CAD build for the part. Positions are in the model's coordinates, mm. Coordinates: 2 decimals unless noted, no trailing zeros. Order: outer loops, then holes, each group sorted by start corner. A loop starts at its lowest first (then second) coordinate and runs counter-clockwise, first axis right, second up. Notation, with made-up numbers: (-31.75, -22) - (-14.75, -22) arc R13 cw to (-14.75, 0) - close; hole circle Ø1 at (41, -24). An arc over 180 degrees is marked (long way). Return JSON: item names as keys, results as strings.
from build123d import *

# Parameters (mm, degrees)
SKETCH2_R           = 9.525
SKETCH2_R_2         = 8.5725
BOSS_EXTRUDE1_DEPTH = 3.175
BOSS_EXTRUDE2_DEPTH = 3.175
BOSS_EXTRUDE3_DEPTH = 10.16
SKETCH5_R           = 1.4351
CUT_EXTRUDE1_DEPTH  = 19.05


with BuildPart() as part:
    # Sketch2 → Boss-Extrude1 (new body, symmetric)
    with BuildSketch(Plane(origin=(0, 0, 0), x_dir=(1, 0, 0), z_dir=(0, 1, 0))):
        Circle(SKETCH2_R)
        Circle(SKETCH2_R_2, mode=Mode.SUBTRACT)
    extrude(amount=BOSS_EXTRUDE1_DEPTH, both=True)

    # Sketch3 → Boss-Extrude2 (add, symmetric)
    with BuildSketch(Plane(origin=(0, 0, 0), x_dir=(1, 0, 0), z_dir=(0, 1, 0))):
        with BuildLine():
            Line((-9.525, 0), (-9.525, -16.764))
            ThreePointArc((-9.525, -16.764), (0, -17.294810057), (9.525, -16.764))
            Line((9.525, -16.764), (9.525, 0))
            ThreePointArc((9.525, 0), (0, -9.525), (-9.525, 0))
        make_face()
    extrude(amount=BOSS_EXTRUDE2_DEPTH, both=True)

    # Sketch4 → Boss-Extrude3 (add)
    with BuildSketch(Plane(origin=(0, 0, 0), x_dir=(1, 0, 0), z_dir=(0, 1, 0))):
        with BuildLine():
            Line((-9.525, -16.764), (-9.525, -13.716))
            Line((-9.525, -13.716), (9.525, -13.716))
            Line((9.525, -13.716), (9.525, -16.764))
            ThreePointArc((9.525, -16.764), (0, -17.294810057), (-9.525, -16.764))
        make_face()
    extrude(amount=BOSS_EXTRUDE3_DEPTH)

    # Sketch5 → Cut-Extrude1 (cut)
    with BuildSketch(Plane(origin=(0, 0, 13.716), x_dir=(-1, 0, 0), z_dir=(0, 0, -1))):
        with Locations((0, 6.6675)):
            Circle(SKETCH5_R)
    extrude(amount=-CUT_EXTRUDE1_DEPTH, mode=Mode.SUBTRACT)


solid = part.part
Item 1: Band-saw the part on A-A, the plane x = 0. List the corners of the cut face in (y, z) (1 decimal), then the cut area to 3 significant figures.
Findings below:
{"outline": "(-3.2, -9.5) - (3.2, -9.5) - (3.2, -8.6) - (-3.2, -8.6) - close; (-3.2, 8.6) - (3.2, 8.6) - (3.2, 13.7) - (5.2, 13.7) - (5.2, 17.3) - (-3.2, 17.3) - close; (8.1, 13.7) - (10.2, 13.7) - (10.2, 17.3) - (8.1, 17.3) - close", "area": "76.2 mm²"}
Item 2: Mould opens along Z. For faces 1 (the cylindrical face through (4.609, -0.044, -7.228)), 2 (the flat face through (0, 5, 13.716)), 3 (the flat face through (0, 3.175, 10)), 4 (the cylindrical face through (-0.134, 3.586, 17.295)) say: released by +Z, released by -Z, zero draft, split by the parting line, or undercut.
Findings below:
{"face 1": "undercut", "face 2": "released by -Z", "face 3": "zero draft", "face 4": "released by +Z"}
Item 3: Band-saw the part on D-D, the plane x = 5. List the corners of the cut face in (y, z) (3 decimals).
Findings below:
{"outline": "(-3.175, -8.107) - (3.175, -8.107) - (3.175, -6.963) - (-3.175, -6.963) - close; (-3.175, 6.963) - (3.175, 6.963) - (3.175, 13.716) - (10.16, 13.716) - (10.16, 17.149) - (-3.175, 17.149) - close"}
Item 4: Band-saw the part on B-B, the plane x = -6. List the corners of the cut face in (y, z) (3 decimals), then the cut area to 3 significant figures.
Findings below:
{"outline": "(-3.175, -7.398) - (3.175, -7.398) - (3.175, -6.123) - (-3.175, -6.123) - close; (-3.175, 6.123) - (3.175, 6.123) - (3.175, 13.716) - (10.16, 13.716) - (10.16, 17.085) - (-3.175, 17.085) - close", "area": "101 mm²"}
Item 5: Wall check: L1, parallel to Z at x = 0, y = -1.25 (1 decimal); L2, parallel to Y at x = 0, z = 16.4 (3 decimals); L3, parallel to X at y = 0.5, z = 0 (1 decimal). Give the ranges that are in metal, low to high. Write a range as [from, to].
Findings below:
{"L1": "z = [-9.5, -8.6], [8.6, 17.3]", "L2": "y = [-3.175, 5.232], [8.103, 10.16]", "L3": "x = [-9.5, -8.6], [8.6, 9.5]"}
Item 6: Drop flat-ended pins along their axis: P1, Ø7.5, axis at x = -4.5, y = 6, coming from the -Z side; P2, Ø3, axis at x = 5.5, y = 7, coming from the -Z side; P3, Ø3, axis at x = -6.5, y = 0.5, coming from the +Z side. Give the stop position or say it passes through.
Findings below:
{"P1": "stops at z = -9.31", "P2": "stops at z = 13.72", "P3": "stops at z = 17.15"}
